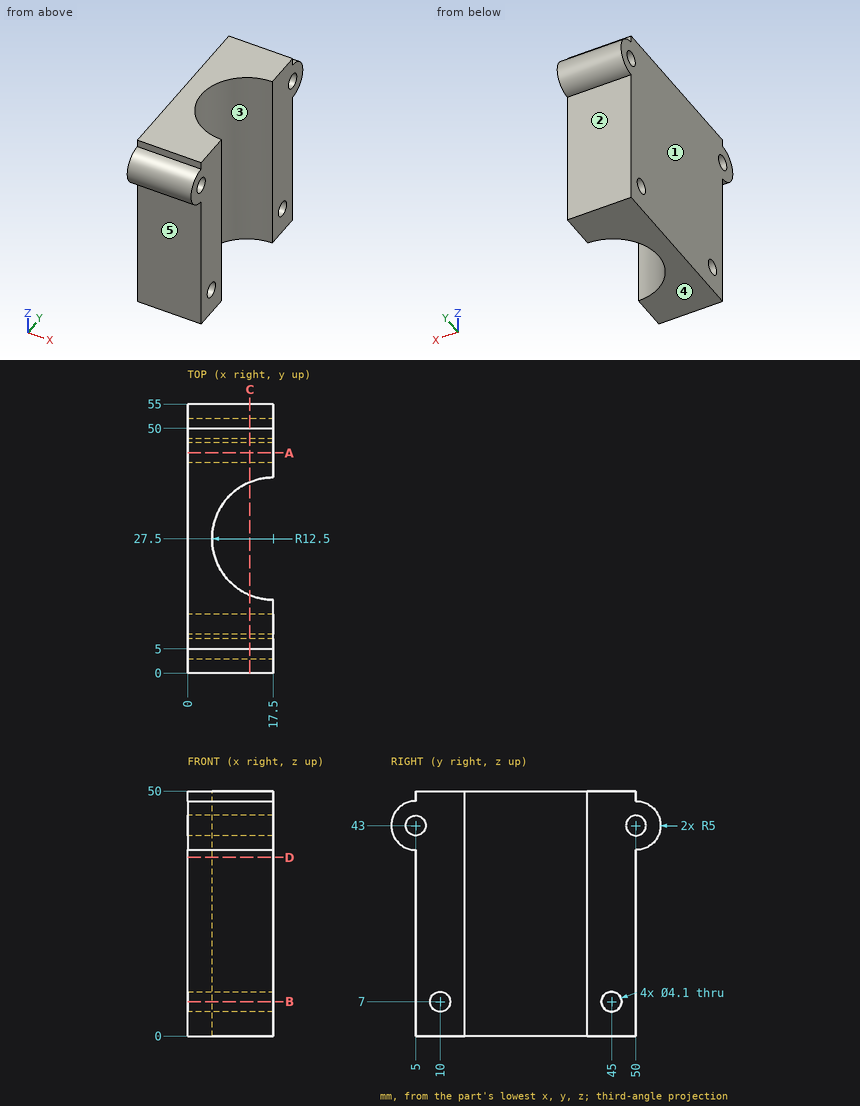
Part print with two shaded views. Sizes in mm from the minimum x, y, z corner. A direction names the side the tool comes from. Coordinates: 2 decimals unless noted, no trailing zeros. Loops run counter-clockwise (first coordinate to the right, second up) from the corner with the lowest first, then second, coordinate; pieces in that order, holes last. Notation, with made-up numbers: M 20,2.25 L 52,2.25 A16 cw 52,24.25 Z; hole C 42,4.25 d11. An arc over 180 degrees is marked long. Use CSV: the item, a comma, the result in double quotes. Start each with the question number.
1. Two-plate mould, pull along Y, no slides. Class the marked faces 3, 4 and 5: pulls with the +Y half, pulls with the -Y half, needs draft (parallel to the pull), parting line crosses it, or undercut.
2. Tool access for the marked faces 1 and 2: list every direction of +Z, -Z, +X, -X, +Y, -Y with a clear straight run to the whole face (end or side of a thin tool).
3. Band-saw the part on B-B, the plane z = 7. List the corners of the cut face in (x, y).
4. Band-saw the part on D-D, the plane z = 36.5. List the corners of the cut face in (x, y), then the cut area to 3 significant figures.
5. Flat gauge pins, fed straight in: pin 1 (1 mm diameter, centred on x = 7.5, z = 49, fed in from +Y); pin 2 (5 mm diameter, centred on x = 13.5, y = 18.5, fed in from +Z); pin 3 (3 mm diameter, centred on x = 10, z = 29.5, fed in from -Y); pin 4 (4 mm diameter, centred on x = 4.5, z = 37, fed in from +Y). Where does each tip first touch, or does it go through?
6. Band-saw the part on A-A, the plane y = 45. List the corners of the cut face in (x, z), then the cut area to 3 significant figures.
7. Band-saw the part on C-C, the plane x = 12.75. List the corners of the cut face in (y, z), then the cut area to 3 significant figures.
8. Probe probe 1 along Y at (x, z) = (4.25, 7); probe 2 along Y at (x, z) = (14.25, 7); probe 3 along Y at (x, z) = (17, 41.5). List the from-to ranges inside material, lowest first. Write a range as [from, to].
Entries:
1,face 3,"undercut"
1,face 4,"needs draft"
1,face 5,"pulls with the -Y half"
2,face 1,"+Z, -Z, -X, +Y, -Y"
2,face 2,"-Z, +X, -X, +Y"
3,outline,"M 0,5 L 17.5,5 L 17.5,7.95 L 0,7.95 Z; M 0,12.05 L 17.5,12.05 L 17.5,15 A12.5 cw 17.5,40 L 17.5,42.95 L 0,42.95 Z; M 0,47.05 L 17.5,47.05 L 17.5,50 L 0,50 Z"
4,outline,"M 0,5 L 17.5,5 L 17.5,15 A12.5 cw 17.5,40 L 17.5,50 L 0,50 Z"
4,area,"542 mm2"
5,pin 1,"stops at y = 50"
5,pin 2,"passes through"
5,pin 3,"stops at y = 5"
5,pin 4,"stops at y = 53"
6,outline,"M 0,0 L 17.5,0 L 17.5,4.95 L 0,4.95 Z; M 0,9.05 L 17.5,9.05 L 17.5,50 L 0,50 Z"
6,area,"803 mm2"
7,outline,"M 5,0 L 15.94,0 L 15.94,50 L 5,50 L 5,48 A5 ccw 5,38 Z; M 39.06,0 L 50,0 L 50,38 A5 ccw 50,48 L 50,50 L 39.06,50 Z; hole C 5,43 d4.1; hole C 10,7 d4.1; hole C 45,7 d4.1; hole C 50,43 d4.1"
7,area,"1,120 mm2"
8,probe 1,"y = [5, 7.95], [12.05, 42.95], [47.05, 50]"
8,probe 2,"y = [5, 7.95], [12.05, 15.43], [39.57, 42.95], [47.05, 50]"
8,probe 3,"y = [0.23, 3.6], [6.4, 15.01], [39.99, 48.6], [51.4, 54.77]"
